The model under review builds one solid part; all positions refer to its coordinate system, in mm. Face numbers are marked on the shaded views. Round coordinates to 2 decimals unless told otherwise and drop trailing zeros. Write each loop counter-clockwise with the first axis right and the second up, starting at its lowest first coordinate (ties: lowest second). Pieces come first, ordered by that corner, then holes. Notation, with made-up numbers: (45.25, 29.25) - (89.25, 29.25) arc R32 cw to (89.25, 56.25) - close; hole circle Ø1 at (81.5, -8.75). An arc over 180 degrees is marked (long way). Return JSON: item names as keys, results as strings.
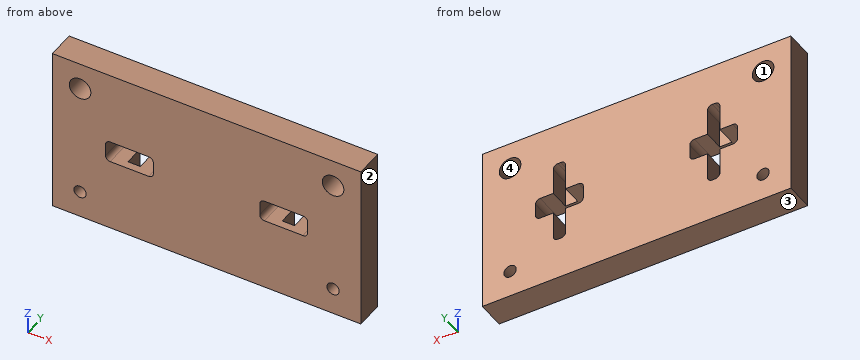
from build123d import *

# Parameters (mm, degrees)
SKETCH1_W           = 200
SKETCH1_H           = 108.68
BOSS_EXTRUDE1_DEPTH = 18
SKETCH2_R           = 4
SKETCH2_R_2         = 7
SKETCH2_W           = 31
SKETCH2_H           = 14
CUT_EXTRUDE1_DEPTH  = 30
SKETCH3_W           = 8
SKETCH3_H           = 20
CUT_EXTRUDE2_DEPTH  = 13
FILLET1_R           = 3


with BuildPart() as part:
    # Sketch1 → Boss-Extrude1 (new body)
    with BuildSketch(Plane(origin=(0, 0, 0), x_dir=(1, 0, 0), z_dir=(0, 1, 0))):
        with Locations((100, -54.34)):
            Rectangle(SKETCH1_W, SKETCH1_H)
    extrude(amount=BOSS_EXTRUDE1_DEPTH)

    # Sketch2 → Cut-Extrude1 (cut)
    with BuildSketch(Plane(origin=(0, 18, 0), x_dir=(1, 0, 0), z_dir=(0, 1, 0))):
        with Locations(Location((18, -17.5, 0), (0, 0, 270))):
            Circle(SKETCH2_R)
        with Locations(Location((182, -17.5, 0), (0, 0, 270))):
            Circle(SKETCH2_R)
        with Locations(Location((18, -91.18, 0), (0, 0, 270))):
            Circle(SKETCH2_R_2)
        with Locations(Location((182, -91.18, 0), (0, 0, 270))):
            Circle(SKETCH2_R_2)
        with Locations((150, -54.34)):
            Rectangle(SKETCH2_W, SKETCH2_H)
        with Locations((50, -54.34)):
            Rectangle(SKETCH2_W, SKETCH2_H)
    extrude(amount=-CUT_EXTRUDE1_DEPTH, mode=Mode.SUBTRACT)

    # Sketch3 → Cut-Extrude2 (cut)
    with BuildSketch(Plane(origin=(0, 18, 0), x_dir=(1, 0, 0), z_dir=(0, 1, 0))):
        with Locations((50, -37.34)):
            Rectangle(SKETCH3_W, SKETCH3_H)
        with Locations((50, -71.34)):
            Rectangle(SKETCH3_W, SKETCH3_H)
        with Locations((150, -71.34)):
            Rectangle(SKETCH3_W, SKETCH3_H)
        with Locations((150, -37.34)):
            Rectangle(SKETCH3_W, SKETCH3_H)
    extrude(amount=-CUT_EXTRUDE2_DEPTH, mode=Mode.SUBTRACT)

    # Fillet1
    fillet1_edges = [part.edges().sort_by_distance(p)[0] for p in [
        (146, 11.5, 27.34),
        (154, 11.5, 27.34),
        (34.5, 9, 61.34),
        (34.5, 9, 47.34),
        (65.5, 9, 47.34),
        (65.5, 9, 61.34),
        (134.5, 9, 47.34),
        (165.5, 9, 47.34),
        (165.5, 9, 61.34),
        (134.5, 9, 61.34),
        (46, 11.5, 27.34),
        (54, 11.5, 27.34),
        (46, 11.5, 81.34),
        (54, 11.5, 81.34),
        (154, 11.5, 81.34),
        (146, 11.5, 81.34),
    ]]
    fillet(fillet1_edges, radius=FILLET1_R)


solid = part.part
(1) Add section C-C (x = 18). Write out the cut boundary in (y, z).
Filled in:
{"outline": "(0, 0) - (18, 0) - (18, 13.5) - (0, 13.5) - close; (0, 21.5) - (18, 21.5) - (18, 84.18) - (0, 84.18) - close; (0, 98.18) - (18, 98.18) - (18, 108.68) - (0, 108.68) - close"}
(2) Add section B-B (z = 91.18). Write out the cut boundary in (x, y).
Filled in:
{"outline": "(0, 0) - (11, 0) - (11, 18) - (0, 18) - close; (25, 0) - (175, 0) - (175, 18) - (25, 18) - close; (189, 0) - (200, 0) - (200, 18) - (189, 18) - close"}
(3) Clearance check with flat-ended pins moving along their axes: pin 1 Ø1.5 at (y, z) = (14, 81.5) entering from -X; pin 2 Ø2.5 at (x, z) = (150.5, 74.5) entering from +Y. State where each tip first meets the part, or that it passes through.
Filled in:
{"pin 1": "stops at x = 0", "pin 2": "stops at y = 5"}
(4) Mouldability with a two-part tool opening along Z and no side actions: class the marked faces 1, 2, 3 and 4 as released by +Z, released by -Z, zero draft, split by the parting line, or undercut.
Filled in:
{"face 1": "undercut", "face 2": "zero draft", "face 3": "released by -Z", "face 4": "undercut"}
(5) Add section D-D (y = 12). Give the number of separate pieces and of enclosed holes in the cut face, plus the area to 3 significant figures.
Filled in:
{"separate pieces": "1", "enclosed holes": "6", "area": "19,900 mm2"}
(6) Add section A-A (x = 160). Write out the cut boundary in (y, z).
Filled in:
{"outline": "(0, 0) - (18, 0) - (18, 47.34) - (0, 47.34) - close; (0, 61.34) - (18, 61.34) - (18, 108.68) - (0, 108.68) - close"}
(7) Wall thickness on line 1 (X direction, y = 6.5, z = 91.18); line 2 (X direction, y = 9.25, z = 52.5); line 3 (Z direction, x = 158.5, y = 8.75): over which ranges is each line inside the solid? List them lowest first.
Filled in:
{"line 1": "x = 0 to 11, 25 to 175, 189 to 200", "line 2": "x = 0 to 34.5, 65.5 to 134.5, 165.5 to 200", "line 3": "z = 0 to 47.34, 61.34 to 108.68"}
